Answer from the drawing. Dimensions are ordinates in mm from the lowest x, y and z of the part. A direction names the side the tool comes from. Round coordinates to 2 decimals unless told otherwise and drop trailing zeros. Order: outer loops, then holes, each group sorted by start corner. A loop starts at its lowest first (then second) coordinate and runs counter-clockwise, first axis right, second up. Notation, with made-up numbers: M 54.25,69.5 L 58.25,69.5 A24 ccw 58.25,107.5 Z; hole C -8,-5.75 d10. An arc over 180 degrees is marked long. Use one line per item in the form item = value. Start each with the question number.
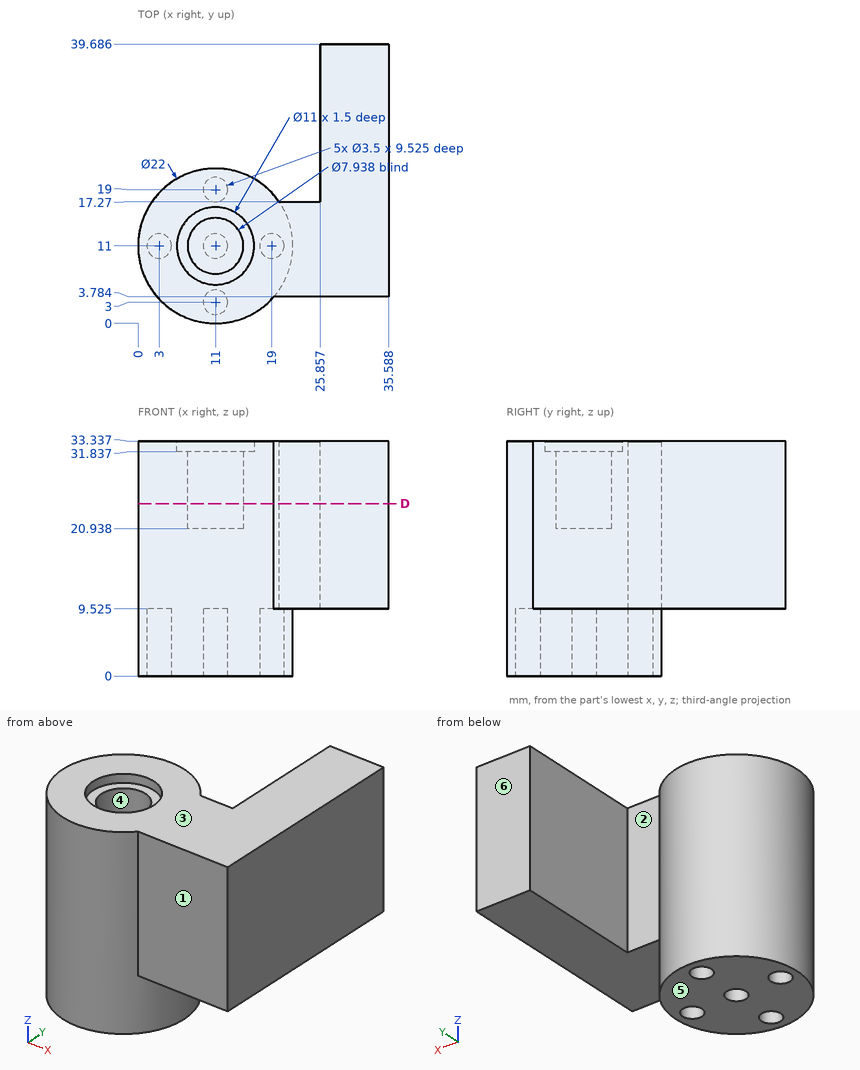
Item 1: For a pull along Y with two mould halves and no side action, classify the marked faces 4, 5 and 6 as pulls with the +Y half, pulls with the -Y half, needs draft (parallel to the pull), parting line crosses it, or undercut.
Item 2: Find the intervals of material crossed by L1, parallel to Y at x = 11, z = 5; L2, parallel to Y at x = 34.5, z = 31.5; L3, parallel to Y at x = 3, z = 2, in increasing order. Write a range as [from, to].
Item 3: Section D-D (z = 24.5) is taken. Write down the section's boundary in (x, y).
Item 4: A tool of negligible diameter and unlimited length cuts with its end or side. For the marked faces 1, 2 and 3, from which of +Z, -Z, +X, -X, +Y, -Y can it reach the whole face along a straight path? Write none if from no direction.
Item 5: Given P1, Ø6.5, axis at x = 13, y = 11.5, coming from the +Z side; P2, Ø18, axis at x = 27, z = 23, coming from the -Y side (1 decimal); P3, Ø5, axis at y = 32.5, z = 16.5, coming from the -X side; P4, Ø8, axis at x = 11, y = 27.5, coming from the +Z side, each flat-ended and moving along its own axis, determine where each tip first touches the part or whether it passes through.
The answers:
q1.face_4 = undercut
q1.face_5 = needs draft
q1.face_6 = pulls with the +Y half
q2.L1 = [0, 1.25], [4.75, 9.25], [12.75, 17.25], [20.75, 22]
q2.L2 = [3.78, 39.69]
q2.L3 = [3.45, 9.25], [12.75, 18.55]
q3.outline = M 19.3,3.78 L 35.59,3.78 L 35.59,39.69 L 25.86,39.69 L 25.86,17.27 L 20.04,17.27 A11 ccw long Z; hole C 11,11 d7.94
q4.face_1 = +Z, -Z, +X, -Y
q4.face_2 = +Z, -Z, +Y
q4.face_3 = +Z, +X, -X, +Y, -Y
q5.P1 = 31.84
q5.P2 = 2.5
q5.P3 = 25.86
q5.P4 = through
